Source: CAD feature listing. Evaluate the final solid. Frame: model axes, mm. Coordinates: 2 decimals unless noted, no trailing zeros. Loops run counter-clockwise (first coordinate to the right, second up) from the corner with the lowest first, then second, coordinate; pieces in that order, holes last.
from build123d import *

# Parameters (mm, degrees)
SKIZZE1_W                       = 92.5
SKIZZE1_H                       = 150
AUFSATZ_LINEAR_AUSTRAGEN1_DEPTH = 2
SCHNITT_LINEAR_AUSTRAGEN1_DEPTH = 177.239184065
LINEARES_MUSTER1_COUNT          = 2
LINEARES_MUSTER1_PITCH          = 30
SPIEGELN1_COPY_1_DEPTH          = 177.239184065
SKIZZE3_W                       = 13.2
SKIZZE3_H                       = 20
SCHNITT_LINEAR_AUSTRAGEN2_DEPTH = 177.239184065
VERRUNDUNG1_R                   = 1
VERRUNDUNG2_R                   = 1
SKIZZE4_W                       = 11.2
SKIZZE4_H                       = 30.8
SCHNITT_LINEAR_AUSTRAGEN3_DEPTH = 177.239184065
VERRUNDUNG3_R                   = 1


with BuildPart() as part:
    # Skizze1 → Aufsatz-Linear austragen1 (new body)
    with BuildSketch(Plane(origin=(0, 0, 0), x_dir=(1, 0, 0), z_dir=(0, 1, 0))):
        with Locations((46.25, 75)):
            Rectangle(SKIZZE1_W, SKIZZE1_H)
    extrude(amount=AUFSATZ_LINEAR_AUSTRAGEN1_DEPTH)

    # Skizze2 → Schnitt-Linear austragen1 (cut, through all)
    with BuildSketch(Plane(origin=(0, 2, 0), x_dir=(1, 0, 0), z_dir=(0, 1, 0))):
        with BuildLine():
            Line((20.8, 130.980352328), (20.8, 125.019647672))
            ThreePointArc((20.8, 125.019647672), (25, 122.85), (29.2, 125.019647672))
            Line((29.2, 125.019647672), (29.2, 130.980352328))
            ThreePointArc((29.2, 130.980352328), (25, 133.15), (20.8, 130.980352328))
        make_face()
    schnitt_linear_austragen1 = extrude(amount=-SCHNITT_LINEAR_AUSTRAGEN1_DEPTH, mode=Mode.SUBTRACT)

    # Lineares Muster1: Schnitt-Linear austragen1 ×2
    with Locations(*[(0, 0, i * LINEARES_MUSTER1_PITCH) for i in range(1, LINEARES_MUSTER1_COUNT)]):
        add(schnitt_linear_austragen1, mode=Mode.SUBTRACT)

    # Spiegeln1: Schnitt-Linear austragen1 across plane
    add(schnitt_linear_austragen1.mirror(Plane(origin=(46.25, 0, 0), x_dir=(0, 0, 1), z_dir=(1, 0, 0))), mode=Mode.SUBTRACT)

    # Spiegeln1 copy 1 sketch → Spiegeln1 copy 1 (cut, through all)
    with BuildSketch(Plane(origin=(92.5, 2, 30), x_dir=(-1, 0, 0), z_dir=(0, 1, 0))):
        with BuildLine():
            Line((20.8, -130.980352328), (20.8, -125.019647672))
            ThreePointArc((20.8, -125.019647672), (25, -122.85), (29.2, -125.019647672))
            Line((29.2, -125.019647672), (29.2, -130.980352328))
            ThreePointArc((29.2, -130.980352328), (25, -133.15), (20.8, -130.980352328))
        make_face()
    extrude(amount=-SPIEGELN1_COPY_1_DEPTH, mode=Mode.SUBTRACT)

    # Skizze3 → Schnitt-Linear austragen2 (cut, through all)
    with BuildSketch(Plane(origin=(0, 2, 0), x_dir=(1, 0, 0), z_dir=(0, 1, 0))):
        with Locations((15.85, 68)):
            Rectangle(SKIZZE3_W, SKIZZE3_H)
        with Locations((56.115, 68)):
            Rectangle(SKIZZE3_W, SKIZZE3_H)
        with Locations((36.385, 68)):
            Rectangle(SKIZZE3_W, SKIZZE3_H)
        with Locations((76.65, 68)):
            Rectangle(SKIZZE3_W, SKIZZE3_H)
    extrude(amount=-SCHNITT_LINEAR_AUSTRAGEN2_DEPTH, mode=Mode.SUBTRACT)

    # Verrundung1
    verrundung1_edges = [part.edges().sort_by_distance(p)[0] for p in [
        (29.785, 1, -58),
        (29.785, 1, -78),
        (42.985, 1, -78),
        (42.985, 1, -58),
        (62.715, 1, -58),
        (49.515, 1, -58),
        (49.515, 1, -78),
        (62.715, 1, -78),
        (83.25, 1, -58),
        (70.05, 1, -58),
        (70.05, 1, -78),
        (83.25, 1, -78),
        (9.25, 1, -58),
        (9.25, 1, -78),
        (22.45, 1, -78),
        (22.45, 1, -58),
    ]]
    fillet(verrundung1_edges, radius=VERRUNDUNG1_R)

    # Verrundung2
    verrundung2_edges = [part.edges().sort_by_distance(p)[0] for p in [
        (20.8, 1, -130.980352328),
        (29.2, 1, -130.980352328),
        (29.2, 1, -125.019647672),
        (20.8, 1, -125.019647672),
        (20.8, 1, -100.980352328),
        (29.2, 1, -100.980352328),
        (29.2, 1, -95.019647672),
        (20.8, 1, -95.019647672),
        (63.3, 1, -130.980352328),
        (71.7, 1, -130.980352328),
        (71.7, 1, -125.019647672),
        (63.3, 1, -125.019647672),
        (63.3, 1, -100.980352328),
        (71.7, 1, -100.980352328),
        (71.7, 1, -95.019647672),
        (63.3, 1, -95.019647672),
    ]]
    fillet(verrundung2_edges, radius=VERRUNDUNG2_R)

    # Skizze4 → Schnitt-Linear austragen3 (cut, through all)
    with BuildSketch(Plane(origin=(0, 2, 0), x_dir=(1, 0, 0), z_dir=(0, 1, 0))):
        with Locations((15.85, 27.6)):
            Rectangle(SKIZZE4_W, SKIZZE4_H)
        with Locations((36.385, 27.6)):
            Rectangle(SKIZZE4_W, SKIZZE4_H)
    schnitt_linear_austragen3 = extrude(amount=-SCHNITT_LINEAR_AUSTRAGEN3_DEPTH, mode=Mode.SUBTRACT)

    # Spiegeln2: Schnitt-Linear austragen3 across plane
    add(schnitt_linear_austragen3.mirror(Plane(origin=(46.25, 0, 0), x_dir=(0, 0, 1), z_dir=(1, 0, 0))), mode=Mode.SUBTRACT)

    # Verrundung3
    verrundung3_edges = [part.edges().sort_by_distance(p)[0] for p in [
        (10.25, 1, -12.2),
        (10.25, 1, -43),
        (21.45, 1, -43),
        (21.45, 1, -12.2),
        (30.785, 1, -12.2),
        (30.785, 1, -43),
        (41.985, 1, -43),
        (41.985, 1, -12.2),
        (82.25, 1, -43),
        (82.25, 1, -12.2),
        (71.05, 1, -12.2),
        (71.05, 1, -43),
        (61.715, 1, -43),
        (61.715, 1, -12.2),
        (50.515, 1, -12.2),
        (50.515, 1, -43),
    ]]
    fillet(verrundung3_edges, radius=VERRUNDUNG3_R)


solid = part.part
Q1. Section B-B, the plane x = 15. Return the cut outline in (y, z).
Q2. Line query: line 1 along Z through (x, y) = (11.5, 1.2); line 2 along X through (y, z) = (1.8, -29.5) (3 decimals); line 3 along Z through (x, y) = (82, 0.8). Output: solid intervals per line, ascending.
Q3. Section A-A, the plane z = -70.5. Return the cut outline in (x, y) (3 decimals).
Q4. Section C-C, the plane z = -36. Return the cut outline in (x, y) (3 decimals), plus the area to 3 significant figures.
Q5. Section D-D, the plane y = 1.7. Count the separate pieces of the cut face and the enclosed holes in it, plus the area to 3 significant figures.
Derived:
1. outline: (0, -150) - (2, -150) - (2, -78) - (0, -78) - close; (0, -58) - (2, -58) - (2, -43) - (0, -43) - close; (0, -12.2) - (2, -12.2) - (2, 0) - (0, 0) - close
2. line 1: z = -150 to -78, -58 to -43, -12.2 to 0
2. line 2: x = 0 to 10.25, 21.45 to 30.785, 41.985 to 50.515, 61.715 to 71.05, 82.25 to 92.5
2. line 3: z = -150 to -78, -58 to -42.66, -12.54 to 0
3. outline: (0, 0) - (9.25, 0) - (9.25, 2) - (0, 2) - close; (22.45, 0) - (29.785, 0) - (29.785, 2) - (22.45, 2) - close; (42.985, 0) - (49.515, 0) - (49.515, 2) - (42.985, 2) - close; (62.715, 0) - (70.05, 0) - (70.05, 2) - (62.715, 2) - close; (83.25, 0) - (92.5, 0) - (92.5, 2) - (83.25, 2) - close
4. outline: (0, 0) - (10.25, 0) - (10.25, 2) - (0, 2) - close; (21.45, 0) - (30.785, 0) - (30.785, 2) - (21.45, 2) - close; (41.985, 0) - (50.515, 0) - (50.515, 2) - (41.985, 2) - close; (61.715, 0) - (71.05, 0) - (71.05, 2) - (61.715, 2) - close; (82.25, 0) - (92.5, 0) - (92.5, 2) - (82.25, 2) - close
4. area: 95.4 mm2
5. separate pieces: 1
5. enclosed holes: 12
5. area: 11,100 mm2
